Build history of the part. All positions in model axes, mm. Face numbers are marked on the shaded views. A direction names the side the tool comes from. Give positions to 0.01 mm unless a question says otherwise; leave off trailing zeros. Order: outer loops, then holes, each group sorted by start corner. A loop starts at its lowest first (then second) coordinate and runs counter-clockwise, first axis right, second up. Notation, with made-up numbers: (-21, 61.25) - (2, 61.25) arc R5 ccw to (2, 68.25) - close; hole circle Ø9 at (-6, 89.25). An arc over 180 degrees is marked (long way). Answer in a Markdown table with one row per item.
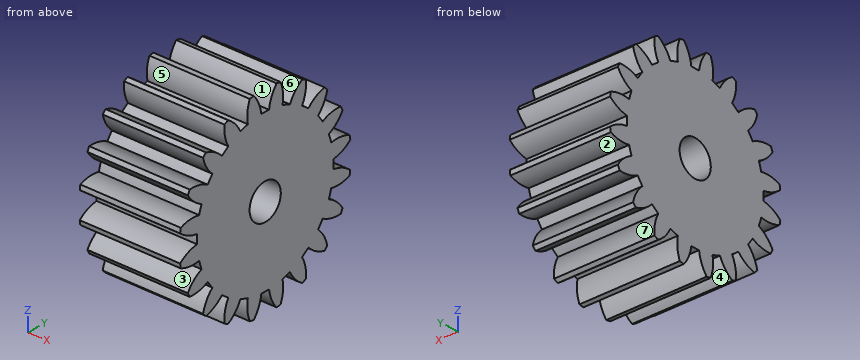
```python
from build123d import *

# Parameters (mm, degrees)
BASPROSKE_W         = 5.7
BASPROSKE_H         = 5.5
TOOTHCUT_DEPTH      = 10.643132271
TEETHCUTS_COUNT     = 20
TEETHCUTS_ANGLE     = 342
BORSKE_R            = 0.4
BORE_DEPTH          = 50.0000508
SKETCH_1_R          = 1
CUT_EXTRUDE_1_DEPTH = 10


with BuildPart() as part:
    # BasProSke → Base-Revolve (revolve)
    with BuildSketch(Plane(origin=(0, 0, 0), x_dir=(1, 0, 0), z_dir=(0, 1, 0)), mode=Mode.PRIVATE) as base_revolve_sk:
        with Locations((2.85, 2.75)):
            Rectangle(BASPROSKE_W, BASPROSKE_H)
    revolve(base_revolve_sk.sketch.rotate(Axis((-10, 0, 0), (1, 0, 0)), 180), axis=Axis((-10, 0, 0), (1, 0, 0)))

    # TooCutSke → ToothCut (cut, through all)
    with BuildSketch(Plane(origin=(0, 0, 0), x_dir=(0, 0, -1), z_dir=(1, 0, 0))):
        with BuildLine():
            ThreePointArc((0.249903181, 4.366855207), (0, 4.374), (-0.249903181, 4.366855207))
            ThreePointArc((-0.249903181, 4.366855207), (-0.415207844, 4.95951031), (-0.752843848, 5.473871692))
            ThreePointArc((-0.752843848, 5.473871692), (0, 5.5254), (0.752843848, 5.473871692))
            ThreePointArc((0.752843848, 5.473871692), (0.415207844, 4.95951031), (0.249903181, 4.366855207))
        make_face()
    toothcut = extrude(amount=TOOTHCUT_DEPTH, mode=Mode.SUBTRACT)

    # TeethCuts: ToothCut ×20 about axis
    teethcuts_axis = Axis((-10, 0, 0), (1, 0, 0))
    for i in range(1, TEETHCUTS_COUNT):
        add(toothcut.rotate(teethcuts_axis, i * TEETHCUTS_ANGLE / (TEETHCUTS_COUNT - 1)), mode=Mode.SUBTRACT)

    # BorSke → Bore (cut, symmetric)
    with BuildSketch(Plane(origin=(0, 0, 0), x_dir=(0, 0, -1), z_dir=(1, 0, 0))):
        with Locations(Location((0, 0, 0), (0, 0, 180))):
            Circle(BORSKE_R)
    extrude(amount=BORE_DEPTH, both=True, mode=Mode.SUBTRACT)

    # 草图1 → 切除-拉伸1 (cut)
    with BuildSketch(Plane(origin=(5.7, 0, 0), x_dir=(0, 0, -1), z_dir=(1, 0, 0))):
        Circle(SKETCH_1_R)
    extrude(amount=-CUT_EXTRUDE_1_DEPTH, mode=Mode.SUBTRACT)


solid = part.part
```
1. Probe line 1 (Y direction, x = 0.25, z = -3.75); line 2 (Z direction, x = 0.95, y = -3.5); line 3 (Y direction, x = 4.95, z = 5). List the from-to ranges inside material, lowest first.
Check result:
| item | result |
|---|---|
| line 1 | y = -3.97 to -3.22, -2.4 to 2.4, 3.22 to 3.97 |
| line 2 | z = -3.89 to -2.88, -2.62 to 2.62, 2.88 to 3.89 |
| line 3 | y = -1.11 to -0.43, 0.43 to 1.11 |
2. Two-plate mould, pull along Z, no slides. Class the marked faces 4, 5, 6 and 7: +Z half, -Z half, draft (parallel to the pull), parting line (faces both ways), or undercut.
Check result:
| item | result |
|---|---|
| face 4 | -Z half |
| face 5 | undercut |
| face 6 | +Z half |
| face 7 | undercut |
3. Drop a flat-ended pin along its axis: P1, Ø2, axis at x = 1, z = 2.5, coming from the -Y side. Give the stop position or say it passes through.
Check result:
| item | result |
|---|---|
| P1 | stops at y = -4.96 |
4. Cut at A-A on y = 0. Write the cut outline in (x, z), and give its area (3 significant figures).
Check result:
| item | result |
|---|---|
| outline | (0, -4.37) - (5.7, -4.37) - (5.7, -1) - (0, -1) - close; (0, 1) - (5.7, 1) - (5.7, 4.37) - (0, 4.37) - close |
| area | 38.5 mm² |
5. Which spindle directions (+Z, -Z, +X, -X, +Y, -Y) get a long thin tool onto all of the face, cutting with end or side? Do the marked faces 1, 2 and 3. Say none if no direction does.
Check result:
| item | result |
|---|---|
| face 1 | +Z, +X, -X |
| face 2 | +X, -X |
| face 3 | +X, -X, -Y |
6. Cut at C-C on z = 2. Write the cut outline in (x, y).
Check result:
| item | result |
|---|---|
| outline | (0, -4.66) - (5.7, -4.66) - (5.7, 4.66) - (0, 4.66) - close |
